Autodesk Inventor part; units mm, degrees
ref_plane "YZ Plane" through (0, 0, 0) normal (1, 0, 0) x (0, 1, 0)
ref_plane "XZ Plane" through (0, 0, 0) normal (0, 1, 0) x (-1, 0, 0)
ref_plane "XY Plane" through (0, 0, 0) normal (0, 0, 1) x (1, 0, 0)
sketch "Boceto2" plane through (0, 0, 0) normal (0, 1, 0) x (-1, 0, 0)
  line L0 (2.5, 5) -> (2.5, 0)
  line L1 (2.5, 0) -> (-2.5, 0)
  line L2 (-2.5, 0) -> (-2.5, 5)
  arc A0 (2.5, 5) -> (-2.5, 5) centre (0, 5) ccw
  circle A1 centre (0, 5) radius 1.2
  point P0 (0, 0)
  point P1 (0, 0)
  dimension "d2" = 5
  dimension "d3" = 5
  dimension "d4" = 2.4
extrude "Extrusión1" add sketch "Boceto2" along normal blind 1.5
sketch "Boceto3" plane through (0, 0, 0) normal (0, 1, 0) x (-1, 0, 0)
  line L0 (-2.5, 1.5) -> (2.5, 1.5)
  line L1 (2.5, 1.5) -> (2.5, 0)
  line L2 (2.5, 0) -> (-2.5, 0)
  line L3 (-2.5, 0) -> (-2.5, 1.5)
  line L4 (-2.5, 0) -> (2.5, 0)
  point P0 (0, 0)
  point P1 (0, 0)
  dimension "d7" = 5
  dimension "d8" = 1.5
extrude "Extrusión2" add sketch "Boceto3" along normal blind 5
fillet "Empalme1" radius 1 1 edges at (0, 1.5, 1.5)
properties part number "support_electronics" material "Plástico ABS"
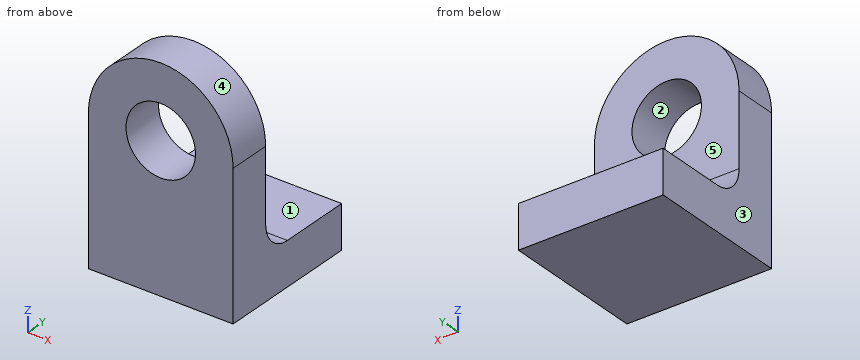
Design review of the part built by this model. Coordinates are the model's own, in mm. Face numbers are marked on the shaded views. A direction names the side the tool comes from. Give positions to 0.01 mm unless a question says otherwise; leave off trailing zeros. Loops run counter-clockwise (first coordinate to the right, second up) from the corner with the lowest first, then second, coordinate; pieces in that order, holes last. Notation, with made-up numbers: (52, 82) - (85, 82) arc R23 cw to (85, 107) - close; hole circle Ø7 at (-22.75, -3). An arc over 180 degrees is marked (long way). Write item = value, one per line.
1) To check wall thickness, follow line 1 (Z direction, x = 0, y = 0.5); line 2 (Y direction, x = 0.55, z = 3.5). State the ranges of each line that lie inside material, in increasing order.
Result sheet:
line_1 = 0 to 3.8, 6.2 to 7.5
line_2 = 0 to 1.5
2) Draft analysis for pull direction X (two halves, no side actions). For the marked faces 1, 2 and 3, state which applies: +X half, -X half, draft (parallel to the pull), parting line (faces both ways), or undercut.
Result sheet:
face_1 = draft
face_2 = undercut
face_3 = -X half
3) Clearance check with flat-ended pins moving along their axes: pin 1 Ø2.5 at (x, z) = (0.5, 4) entering from +Y; pin 2 Ø1.5 at (x, y) = (-1, 1.5) entering from +Z; pin 3 Ø3 at (x, y) = (0.5, 4) entering from +Z. State where each tip first meets the part, or that it passes through.
Result sheet:
pin_1 = 1.5
pin_2 = 7.49
pin_3 = 1.5
4) Take a section at C-C on z = 4.75. State the section outline as (x, y) points, and give its area (3 significant figures).
Result sheet:
outline = (-2.5, 0) - (-1.17, 0) - (-1.17, 1.5) - (-2.5, 1.5) - close; (1.17, 0) - (2.5, 0) - (2.5, 1.5) - (1.17, 1.5) - close
area = 3.98 mm2
5) Take a section at B-B on y = 1.1. State the section outline as (x, z) points.
Result sheet:
outline = (-2.5, 0) - (2.5, 0) - (2.5, 5) arc R2.5 ccw to (-2.5, 5) - close; hole circle Ø2.4 at (0, 5)
6) Take a section at A-A on x = 0. State the section outline as (y, z) points.
Result sheet:
outline = (0, 0) - (5, 0) - (5, 1.5) - (2.5, 1.5) arc R1 cw to (1.5, 2.5) - (1.5, 3.8) - (0, 3.8) - close; (0, 6.2) - (1.5, 6.2) - (1.5, 7.5) - (0, 7.5) - close
7) Tool access review of the marked faces 4 and 5: name each direction out of +Z, -Z, +X, -X, +Y, -Y from which nothing blocks a thin tool from reaching the whole face with its end or side.
Result sheet:
face_4 = +Z, +Y, -Y
face_5 = +Z, +X, -X, +Y
8) Take a section at D-D on x = 0.65. State the section outline as (y, z) points.
Result sheet:
outline = (0, 0) - (5, 0) - (5, 1.5) - (2.5, 1.5) arc R1 cw to (1.5, 2.5) - (1.5, 3.99) - (0, 3.99) - close; (0, 6.01) - (1.5, 6.01) - (1.5, 7.41) - (0, 7.41) - close
